Could you check a few things on this model? Use its own coordinates, in mm. A direction names the side the tool comes from. Coordinates: 2 decimals unless noted, no trailing zeros. Loops run counter-clockwise (first coordinate to the right, second up) from the corner with the lowest first, then second, coordinate; pieces in that order, holes last. Notation, with made-up numbers: M 19.25,-10.5 L 42.25,-10.5 A16 cw 42.25,-4.5 Z; hole C 82,-34 d3. An arc over 180 degrees is marked long. Write each question's results on one line, items separated by ' | '.
Autodesk Inventor part; units mm, degrees
ref_plane "Work Plane1" through (83.5, 0, -139.5) normal (1, 0, 0) x (0, 0, -1)
ref_plane "YZ Plane" through (0, 0, 0) normal (1, 0, 0) x (0, 1, 0)
ref_plane "XZ Plane" through (0, 0, 0) normal (0, 1, 0) x (-1, 0, 0)
sketch "Sketch1" plane through (0, 0, 0) normal (0, 1, 0) x (-1, 0, 0)
  line L0 (-83.5, 139.5) -> (83.5, 139.5)
  line L1 (83.5, 139.5) -> (83.5, -139.5)
  line L2 (83.5, -139.5) -> (-83.5, -139.5)
  line L3 (-83.5, -139.5) -> (-83.5, 139.5)
  line L4 (-83.5, 139.5) -> (83.5, -139.5) construction
  line L5 (83.5, 139.5) -> (-83.5, -139.5) construction
  point P0 (0, 0)
  dimension "d0" = 167
  dimension "d1" = 279
extrude "Extrusion1" add sketch "Sketch1" along normal blind 13.4
sketch "Sketch2" plane through (0, 13.4, 0) normal (0, 1, 0) x (1, 0, 0)
  line L0 (72.25, -115.05) -> (-72.25, -115.05)
  line L1 (-72.25, -115.05) -> (-72.25, 115.05)
  line L2 (-72.25, 115.05) -> (72.25, 115.05)
  line L3 (72.25, 115.05) -> (72.25, -115.05)
  line L4 (72.25, -115.05) -> (-72.25, 115.05) construction
  line L5 (-72.25, -115.05) -> (72.25, 115.05) construction
  point P0 (0, 0)
  dimension "d4" = 144.5
  dimension "d5" = 230.1
extrude "Extrusion2" cut sketch "Sketch2" against normal blind 8.4
sketch "Sketch4" plane through (0, 13.4, 0) normal (0, 1, 0) x (1, 0, 0)
  circle A0 centre (-77.5, -133.5) radius 1.25
  line L0 (-83.5, 139.5) -> (-83.5, -139.5)
  line L1 (-83.5, -139.5) -> (83.5, -139.5)
  circle A1 centre (-77.5, 133.5) radius 1.25
  line L2 (83.5, 139.5) -> (-83.5, 139.5)
  circle A2 centre (77.5, 133.5) radius 1.25
  line L3 (83.5, -139.5) -> (83.5, 139.5)
  circle A3 centre (77.5, -133.5) radius 1.25
  point P0 (0, 0)
  dimension "d16" = 2.5
  dimension "d17" = 6
  dimension "d18" = 6
  dimension "d19" = 2.5
  dimension "d20" = 6
  dimension "d21" = 6
  dimension "d22" = 2.5
  dimension "d23" = 6
  dimension "d24" = 6
  dimension "d25" = 2.5
  dimension "d26" = 6
  dimension "d27" = 6
extrude "Extrusion4" cut sketch "Sketch4" against normal through all contours A0 | A1 | A2 | A3
sketch "Sketch5" plane through (0, 13.4, 0) normal (0, 1, 0) x (1, 0, 0)
  line L0 (-72.25, -115.05) -> (-72.25, 115.05)
  line L1 (72.25, -115.05) -> (-72.25, -115.05)
  line L2 (-77.25, -120.05) -> (-72.25, -120.05)
  line L3 (-72.25, -120.05) -> (-72.25, 120.05)
  line L4 (-72.25, 120.05) -> (-77.25, 120.05)
  line L5 (-77.25, 120.05) -> (-77.25, -120.05)
  line L6 (72.25, 115.05) -> (72.25, -115.05)
  line L7 (77.25, -120.05) -> (72.25, -120.05)
  line L8 (72.25, -120.05) -> (72.25, 120.05)
  line L9 (72.25, 120.05) -> (77.25, 120.05)
  line L10 (77.25, 120.05) -> (77.25, -120.05)
  line L11 (-72.25, 115.05) -> (72.25, 115.05)
  line L12 (72.25, 120.05) -> (-72.25, 120.05)
  line L13 (-72.25, 120.05) -> (-72.25, 115.05)
  line L14 (-72.25, 115.05) -> (72.25, 115.05)
  line L15 (72.25, 115.05) -> (72.25, 120.05)
  line L16 (-72.25, -115.05) -> (72.25, -115.05)
  line L17 (72.25, -115.05) -> (72.25, -120.05)
  line L18 (72.25, -120.05) -> (-72.25, -120.05)
  line L19 (-72.25, -120.05) -> (-72.25, -115.05)
  point P0 (0, 0)
  dimension "d30" = 5
  dimension "d31" = 5
  dimension "d32" = 240.1
  dimension "d33" = 5
  dimension "d34" = 5
  dimension "d35" = 240.1
extrude "Extrusion5" add sketch "Sketch5" along normal blind 10 contours L3 L2 L5 L4 L0 | L1 L8 L18 L3 | L3 L12 L8 L11 | L6 L8 L9 L10 L7
sketch "Sketch7" plane through (0, 0, 0) normal (0, -1, 0) x (1, 0, 0)
  circle A0 centre (-77.5, -133.5) radius 1.25
  circle A1 centre (-77.5, -133.5) radius 1.75
  circle A2 centre (-77.5, 133.5) radius 1.25
  circle A3 centre (-77.5, 133.5) radius 1.75
  circle A4 centre (77.5, 133.5) radius 1.25
  circle A5 centre (77.5, 133.5) radius 1.75
  circle A6 centre (77.5, -133.5) radius 1.25
  circle A7 centre (77.5, -133.5) radius 1.75
  point P0 (0, 0)
  dimension "d42" = 3.5
  dimension "d43" = 3.5
  dimension "d44" = 3.5
  dimension "d45" = 3.5
extrude "Extrusion6" cut sketch "Sketch7" against normal blind 11.4 contours A0 | A1 | A2 | A3 | A4 | A5 | A7
sketch "Sketch8" plane through (83.5, 0, 139.5) normal (1, 0, 0) x (0, 0, -1)
  line L0 (139.5, 0) -> (139.5, 13.4)
  line L1 (0, 13.4) -> (279, 13.4)
sketch "Sketch9" plane through (0, 13.4, 0) normal (0, 1, 0) x (1, 0, 0)
  line L0 (83.5, -139.5) -> (83.5, 139.5)
  line L1 (83.5, 0) -> (77.25, 0)
  line L2 (77.25, 120.05) -> (77.25, -120.05)
  point P0 (0, 0)
sketch "Sketch10" plane through (77.25, 13.4, 120.05) normal (1, 0, 0) x (0, 0, -1)
  line L0 (-19.45, 0) -> (259.55, 0)
  line L1 (120.05, 0) -> (120.05, 10)
  line L2 (0, 10) -> (240.1, 10)
  point P0 (120.05, -13.4)
split_face "Split1"
split_face "Split2"
split_face "Split3"
ref_plane "Work Plane1" through (83.5, 0, -139.5) normal (1, 0, 0) x (0, 0, -1)
sketch "Sketch11" plane through (83.5, 0, -139.5) normal (1, 0, 0) x (0, 0, -1)
  line L0 (0, 0) -> (0, 13.4)
  line L1 (-139.5, 5) -> (-139.5, 23.4)
  line L2 (0, 0) -> (-139.5, 0)
  line L3 (-139.5, 0) -> (-139.5, 23.4)
  line L4 (-139.5, 23.4) -> (0, 23.4)
  line L5 (0, 23.4) -> (0, 0)
  line L6 (-279, 0) -> (-139.5, 0)
  line L7 (-259.55, 23.4) -> (-139.5, 23.4)
  line L8 (-279, 0) -> (-139.5, 0)
  line L9 (-139.5, 0) -> (-139.5, 23.4)
  line L10 (-139.5, 23.4) -> (-279, 23.4)
  line L11 (-279, 23.4) -> (-279, 0)
extrude "Extrusion7" cut sketch "Sketch11" against normal blind 167.1625 contours L6 L11 L10 L7 L1 L3
sketch "Sketch12" plane through (-83.5, 0, 0) normal (0, 0, 1) x (1, 0, 0)
  line L0 (0, 0) -> (0, 13.4)
  line L1 (11.25, 5) -> (11.25, 23.4)
  circle A0 centre (5.625, 6.7) radius 2.5
  line L2 (167, 0) -> (167, 13.4)
  circle A1 centre (161.375, 6.7) radius 2.5
  line L3 (11.25, 5) -> (155.75, 5)
  circle A2 centre (58.5, 2.5) radius 1.5
  circle A3 centre (33.5, 2.5) radius 1.5
  circle A4 centre (108.5, 2.5) radius 1.5
  circle A5 centre (133.5, 2.5) radius 1.5
  point P0 (83.5, 0)
  dimension "d51" = 5
  dimension "d53" = 5
  dimension "d55" = 3
  dimension "d57" = 3
  dimension "d59" = 3
  dimension "d61" = 3
extrude "Extrusion8" cut sketch "Sketch12" against normal blind 15
properties part number "Enclosure 2 Bottom" material "ABS Plastic"
(1) Imagine slicing it at A-A, the plane y = 18.5. List the corners of the cut face in (x, z) for me.
Reported:
outline: M -77.25,-120.05 L 77.25,-120.05 L 77.25,0 L 72.25,0 L 72.25,-115.05 L -72.25,-115.05 L -72.25,0 L -77.25,0 Z
(2) Please list where these lines run through material, in increasing order: probe 1 along X at (y, z) = (7.5, -133.5); probe 2 along Y at (x, z) = (-50, -5.5); probe 3 along X at (y, z) = (16.5, -75.5). Write a range as from..to.
Reported:
probe 1: x = -83.5..-79.25, -75.75..75.75, 79.25..83.5 | probe 2: y = 0..1, 4..5 | probe 3: x = -77.25..-72.25, 72.25..77.25
(3) Imagine slicing it at D-D, the plane z = -124.5. List the corners of the cut face in (x, y) for me.
Reported:
outline: M -83.5,0 L 83.5,0 L 83.5,13.4 L -83.5,13.4 Z
(4) Imagine slicing it at C-C, the plane z = -89. List the corners of the cut face in (x, y) for me, and give its area (3 significant figures).
Reported:
outline: M -83.5,0 L 83.5,0 L 83.5,13.4 L 77.25,13.4 L 77.25,23.4 L 72.25,23.4 L 72.25,5 L -72.25,5 L -72.25,23.4 L -77.25,23.4 L -77.25,13.4 L -83.5,13.4 Z | area: 1,120 mm2
(5) If we mould it in two halves opening along X, with no side actions, what happens to faces 5 (the flat face through (-72.25, 14, -57)), 6 (the flat face through (77.25, 18, -61)), 7 (the flat face through (1, 4, 0))? For each: released by +X, released by -X, zero draft, split by the parting line, or undercut.
Reported:
face 5: undercut | face 6: released by +X | face 7: zero draft
(6) Imagine slicing it at B-B, the plane x = -41. List the corners of the cut face in (y, z) for me, and give its area (3 significant figures).
Reported:
outline: M 0,-139.5 L 13.4,-139.5 L 13.4,-120.05 L 23.4,-120.05 L 23.4,-115.05 L 5,-115.05 L 5,0 L 0,0 Z | area: 953 mm2
(7) Will these pins go through, and if not, where does the flat tip stop? P1, Ø2.5, axis at x = 77, y = 6, coming from the +Z side; P2, Ø3, axis at x = 77.5, z = -133.5, coming from the +Y side; P3, Ø6, axis at x = 6.5, z = -27, coming from the +Y side.
Reported:
P1: stops at z = -15 | P2: stops at y = 13.4 | P3: stops at y = 5
(8) Which directions (+Z, -Z, +X, -X, +Y, -Y) give clear straight access to the entire face, cutting with the end or side of a thin tool? Please do faces 1 (the flat face through (76, 11.4, -133)), 2 (the flat face through (-1, 14, -115.05)), 3 (the cylindrical face through (-79.86, 5.18, -7.4)), 4 (the flat face through (1, 18, -120.05)).
Reported:
face 1: -Y | face 2: +Z, +Y | face 3: +Z | face 4: -Z, +X, -X, +Y
